Work out the finished part from the listing and answer in its coordinate system (mm). Face numbers are marked on the shaded views. A direction names the side the tool comes from. Coordinates: 2 decimals unless noted, no trailing zeros. Loops run counter-clockwise (first coordinate to the right, second up) from the corner with the lowest first, then second, coordinate; pieces in that order, holes last. Notation, with made-up numbers: (47.5, 25) - (51.5, 25) arc R37 ccw to (51.5, 63) - close; hole circle Ø7 at (47, -32). An arc over 180 degrees is marked (long way). Write each question's results on one line, items separated by ' | '. Start each with the question number.
1. Which of the six approach directions +Z, -Z, +X, -X, +Y, -Y give full straight-line access (tool end or side, diameter ignored) to the marked faces 1 and 2?
2. Each of these flat-tipped pins is pushed along its axis until it touches: P1, Ø1.5, axis at x = 22.5, y = 44.5, coming from the +Z side; P2, Ø1, axis at x = 25.5, y = 47.5, coming from the -Z side; P3, Ø5, axis at y = 44, z = 6, coming from the +X side; P4, Ø3.5, axis at y = 20, z = 11, coming from the +X side. Where does it stop, or does it pass through?
3. A cutting plane is placed at D-D on y = 51.75. Determine the outline of the cut face in (x, z), then the cut area to 3 significant figures.
4. A cutting plane is placed at B-B on x = 20.5. Determine the outline of the cut face in (y, z).
5. A cutting plane is placed at C-C on z = 4. Determine the outline of the cut face in (x, y), then the cut area to 3 significant figures.
6. Find the intervals of material crossed by line 1 along X through (y, z) = (2.25, 12.3); line 2 along X through (y, z) = (51.75, 12.2); line 3 along Y through (x, z) = (15, 12.4), in increasing order. Write a range as [from, to].
7. A cutting plane is placed at A-A on y = 14.3. Determine the outline of the cut face in (x, z).
from build123d import *

# Parameters (mm, degrees)
SKETCH_1_W          = 3
SKETCH_1_H          = 54
EXTRUDE_1_DEPTH     = 13
SKETCH_3_R          = 1.5
CUT_EXTRUDE_1_DEPTH = 56.623735941
SKETCH_4_W          = 3
SKETCH_4_H          = 54
EXTRUDE_2_DEPTH     = 27
SKETCH_5_W          = 20
SKETCH_5_H          = 40
CUT_EXTRUDE_2_DEPTH = 64.126856408
SKETCH_6_R          = 2.5
SKETCH_6_R_2        = 2.424949467
SKETCH_6_R_3        = 2.447616221
CUT_EXTRUDE_3_DEPTH = 63.577951389


with BuildPart() as part:
    # 草图1 → 凸台-拉伸1 (new body)
    with BuildSketch(Plane.XY):
        with Locations((1.5, 27)):
            Rectangle(SKETCH_1_W, SKETCH_1_H)
    extrude(amount=EXTRUDE_1_DEPTH)

    # 草图3 → 切除-拉伸1 (cut, through all)
    with BuildSketch(Plane(origin=(3, 0, 0), x_dir=(0, 0, -1), z_dir=(1, 0, 0))):
        with Locations((-4, 40.5)):
            Circle(SKETCH_3_R)
        with Locations((-4, 14.3)):
            Circle(SKETCH_3_R)
    extrude(amount=-CUT_EXTRUDE_1_DEPTH, mode=Mode.SUBTRACT)

    # 草图4 → 凸台-拉伸2 (add)
    with BuildSketch(Plane(origin=(3, 0, 0), x_dir=(0, 0, -1), z_dir=(1, 0, 0))):
        with Locations((-11.5, 27)):
            Rectangle(SKETCH_4_W, SKETCH_4_H)
    extrude(amount=EXTRUDE_2_DEPTH)

    # 草图5 → 切除-拉伸2 (cut, through all)
    with BuildSketch(Plane.XY.offset(13)):
        with Locations((20, 27)):
            Rectangle(SKETCH_5_W, SKETCH_5_H)
    extrude(amount=-CUT_EXTRUDE_2_DEPTH, mode=Mode.SUBTRACT)

    # 草图6 → 切除-拉伸3 (cut, through all)
    with BuildSketch(Plane(origin=(0, 0, 10), x_dir=(-1, 0, 0), z_dir=(0, 0, -1))):
        with Locations((-25, 51.75)):
            Circle(SKETCH_6_R)
        with Locations((-25, 2.25)):
            Circle(SKETCH_6_R_2)
        with Locations((-15, 51.75)):
            Circle(SKETCH_6_R_3)
        with Locations((-15, 2.25)):
            Circle(SKETCH_6_R)
    extrude(amount=-CUT_EXTRUDE_3_DEPTH, mode=Mode.SUBTRACT)


solid = part.part
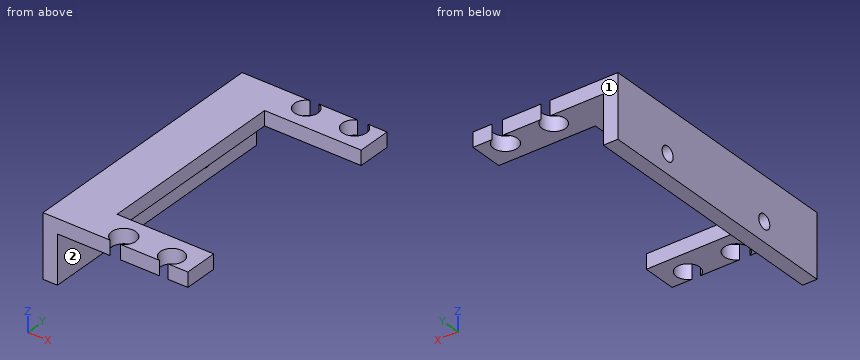
Values:
1) face 1: +Z, -Z, +X, -X, +Y | face 2: -Z, +X, +Y, -Y
2) P1: through | P2: z = 10 | P3: x = 3 | P4: x = 10
3) outline: (0, 0) - (3, 0) - (3, 10) - (12.55, 10) - (12.55, 13) - (0, 13) - close; (17.45, 10) - (22.5, 10) - (22.5, 13) - (17.45, 13) - close; (27.5, 10) - (30, 10) - (30, 13) - (27.5, 13) - close | area: 90.3 mm^2
4) outline: (0, 10) - (7, 10) - (7, 13) - (0, 13) - close; (47, 10) - (54, 10) - (54, 13) - (47, 13) - close
5) outline: (0, 0) - (3, 0) - (3, 12.8) - (0, 12.8) - close; (0, 15.8) - (3, 15.8) - (3, 39) - (0, 39) - close; (0, 42) - (3, 42) - (3, 54) - (0, 54) - close | area: 144 mm^2
6) line 1: [0, 12.5], [17.5, 22.58], [27.42, 30] | line 2: [0, 12.55], [17.45, 22.5], [27.5, 30] | line 3: [4.75, 7], [47, 49.3]
7) outline: (0, 0) - (3, 0) - (3, 2.5) - (0, 2.5) - close; (0, 5.5) - (3, 5.5) - (3, 10) - (10, 10) - (10, 13) - (0, 13) - close
